from build123d import *

# Parameters (mm, degrees)
F0_W     = 90
F0_H     = 70
F0_W_2   = 80
F0_H_2   = 60
F1_DEPTH = 25
F0_R     = 7.5
F2_DEPTH = 5
F0_R_2   = 2.8629120086
F3_DEPTH = 10
F4_R     = 5
F5_SIZE  = 2


with BuildPart() as f1:
    # F0 (on Top) → F1 (new body)
    with BuildSketch(Plane.XY):
        Rectangle(F0_W, F0_H)
        Rectangle(F0_W_2, F0_H_2, mode=Mode.SUBTRACT)
    extrude(amount=F1_DEPTH)

    # F0 (on Top) → F2 (join)
    with BuildSketch(Plane.XY):
        Rectangle(F0_W_2, F0_H_2)
        with Locations((-25, -15)):
            Circle(F0_R, mode=Mode.SUBTRACT)
        with Locations((25, -15)):
            Circle(F0_R, mode=Mode.SUBTRACT)
        with Locations((-25, 15)):
            Circle(F0_R, mode=Mode.SUBTRACT)
        with Locations((25, 15)):
            Circle(F0_R, mode=Mode.SUBTRACT)
    extrude(amount=F2_DEPTH)

    # F0 (on Top) → F3 (join)
    with BuildSketch(Plane.XY):
        with Locations((-25, 15)):
            Circle(F0_R)
        with Locations((-25, 15)):
            Circle(F0_R_2, mode=Mode.SUBTRACT)
        with Locations((-25, -15)):
            Circle(F0_R)
        with Locations((-25, -15)):
            Circle(F0_R_2, mode=Mode.SUBTRACT)
        with Locations((25, 15)):
            Circle(F0_R)
        with Locations((25, 15)):
            Circle(F0_R_2, mode=Mode.SUBTRACT)
        with Locations((25, -15)):
            Circle(F0_R)
        with Locations((25, -15)):
            Circle(F0_R_2, mode=Mode.SUBTRACT)
    extrude(amount=F3_DEPTH)

    # F4
    f4_edges = [f1.edges().sort_by_distance(p)[0] for p in [
        (-40, 30, 15),
        (45, 35, 12.5),
        (45, -35, 12.5),
        (-45, -35, 12.5),
        (-45, 35, 12.5),
        (40, -30, 15),
        (-40, -30, 15),
        (40, 30, 15),
    ]]
    fillet(f4_edges, radius=F4_R)

    # F5
    f5_edges = [f1.edges().sort_by_distance(p)[0] for p in [
        (-32.5, 15, 5),
        (17.5, 15, 5),
        (-32.5, -15, 5),
        (0, -30, 5),
        (-38.535534, -28.535534, 5),
        (38.535534, -28.535534, 5),
        (-40, 0, 5),
        (40, 0, 5),
        (-38.535534, 28.535534, 5),
        (38.535534, 28.535534, 5),
        (0, 30, 5),
        (17.5, -15, 5),
    ]]
    chamfer(f5_edges, length=F5_SIZE)


solid = f1.part
Can you work these out from the model? Positions are in its coordinate system, mm. A direction names the side the tool comes from. Coordinates: 2 decimals unless noted, no trailing zeros. Write each loop counter-clockwise with the first axis right and the second up, starting at its lowest first coordinate (ties: lowest second). Pieces come first, ordered by that corner, then holes. Notation, with made-up numbers: (-4, 45.5) - (54, 45.5) arc R20 cw to (54, 65.5) - close; hole circle Ø5 at (62.5, 0). An arc over 180 degrees is marked (long way). Return JSON: item names as keys, results as strings. Group by question number.
Item 1: I'm going to push flat-ended pins straight in: pin 1 Ø16.5 at (x, y) = (-25.5, 14) entering from +Z; pin 2 Ø3.5 at (x, y) = (25, -15) entering from -Z; pin 3 Ø8 at (x, y) = (23.5, 2.5) entering from +Z. Where does each tip first touch, or does it pass through?
Item 2: If we section it at D-D (x = 10): Write out the boundary of the cut face in (y, z).
Item 3: If we section it at C-C (z = 3.25): Write out the boundary of the cut face in (x, y), then the cut area to 3 significant figures.
Item 4: If we section it at A-A (x = 25): Count the separate pieces of the cut face and the enclosed holes in it, then the cut area to 3 significant figures.
Item 5: Please list where these lines run through material, in increasing order: probe 1 along Y at (x, z) = (-25, 4.25); probe 2 along X at (y, z) = (29, 23); probe 3 along Y at (x, z) = (17, 21).
Item 6: We'd pull the mould along Y, two halves only. Please class faces 1 (the face through (-1, 35, 12)), 2 (the face through (0, 30, 16)), 3 (the face through (-44, -33, 13)): pulls with the +Y half, pulls with the -Y half, needs draft (parallel to the pull), parting line crosses it, or undercut.
Item 7: Which directions (+Z, -Z, +X, -X, +Y, -Y) give clear straight access to the entire face, cutting with the end or side of a thin tool? Please do faces 4 (the face through (28.2, -14.9, 10)), 5 (the face through (-45, 0, 12)).
Return value:
{
 "1": {"pin 1": "stops at z = 10", "pin 2": "passes through", "pin 3": "stops at z = 5.91"},
 "2": {"outline": "(-35, 0) - (35, 0) - (35, 25) - (30, 25) - (30, 7) - (28, 5) - (-28, 5) - (-30, 7) - (-30, 25) - (-35, 25) - close"},
 "3": {"outline": "(-45, -30) arc R5 ccw to (-40, -35) - (40, -35) arc R5 ccw to (45, -30) - (45, 30) arc R5 ccw to (40, 35) - (-40, 35) arc R5 ccw to (-45, 30) - close; hole circle Ø5.73 at (-25, -15); hole circle Ø5.73 at (-25, 15); hole circle Ø5.73 at (25, -15); hole circle Ø5.73 at (25, 15)", "area": "6,180 mm^2"},
 "4": {"separate pieces": "3", "enclosed holes": "0", "area": "597 mm^2"},
 "5": {"probe 1": "y = -35 to -17.86, -12.14 to 12.14, 17.86 to 35", "probe 2": "x = -45 to -38, 38 to 45", "probe 3": "y = -35 to -30, 30 to 35"},
 "6": {"face 1": "pulls with the +Y half", "face 2": "undercut", "face 3": "pulls with the -Y half"},
 "7": {"face 4": "+Z", "face 5": "+Z, -Z, -X, +Y, -Y"}
}
